```python
from build123d import *

# Parameters (mm, degrees)
F0_W     = 152.4
F0_H     = 152.4
F0_R     = 5.159375
F0_R_2   = 6.35
F0_R_3   = 44.45
F1_DEPTH = 12.7


with BuildPart() as f1:
    # F0 (on Top) → F1 (new body)
    with BuildSketch(Plane.XY):
        Rectangle(F0_W, F0_H)
        with Locations((0, -62.4967)):
            Circle(F0_R, mode=Mode.SUBTRACT)
        with Locations((45.960951, -45.960951)):
            Circle(F0_R_2, mode=Mode.SUBTRACT)
        with Locations((-62.4967, 0)):
            Circle(F0_R, mode=Mode.SUBTRACT)
        with Locations((-45.960951, 45.960951)):
            Circle(F0_R_2, mode=Mode.SUBTRACT)
        Circle(F0_R_3, mode=Mode.SUBTRACT)
        with Locations((62.4967, 0)):
            Circle(F0_R, mode=Mode.SUBTRACT)
        with Locations((0, 62.4967)):
            Circle(F0_R, mode=Mode.SUBTRACT)
    extrude(amount=F1_DEPTH)


solid = f1.part
```
Design review of the part built by this model. Coordinates are the model's own, in mm. Coordinates: 2 decimals unless noted, no trailing zeros. Order: outer loops, then holes, each group sorted by start corner. A loop starts at its lowest first (then second) coordinate and runs counter-clockwise, first axis right, second up. Notation, with made-up numbers: (31, -9) -> (75, -9) arc R24 cw to (75, 19) -> close; hole circle Ø10 at (63, -4). An arc over 180 degrees is marked (long way). One line per item, written item: value. Start each with the question number.
Q1. Take a section at D-D, the plane z = 6.5. State the section outline as (x, y) points, then the cut area to 3 significant figures.
Q2. Mouldability with a two-part tool opening along Y and no side actions: class faces 1 (the cylindrical face through (-0.67, -57.38, 6.26)), 2 (the flat face through (-1, 76.2, 6)), 3 (the cylindrical face through (42.397, 13.352, 6.261)), 4 (the flat face through (-35, 35, 12.7)) as pulls with the +Y half, pulls with the -Y half, needs draft (parallel to the pull), parting line crosses it, or undercut.
Q3. Take a section at A-A, the plane y = 0. State the section outline as (x, z) points.
Q4. Take a section at B-B, the plane x = 23.5. State the section outline as (y, z) points.
Q5. For probe 1 along Y at (x, z) = (0, 9); probe 2 along Y at (x, z) = (3, 10.75); probe 3 along Y at (x, z) = (41, 9.25), list the stretches that pass through material, from the lowest coordinate up.
Values follow:
1. outline: (-76.2, -76.2) -> (76.2, -76.2) -> (76.2, 76.2) -> (-76.2, 76.2) -> close; hole circle Ø10.32 at (-62.5, 0); hole circle Ø12.7 at (-45.96, 45.96); hole circle Ø88.9 at (0, 0); hole circle Ø10.32 at (0, -62.5); hole circle Ø10.32 at (0, 62.5); hole circle Ø12.7 at (45.96, -45.96); hole circle Ø10.32 at (62.5, 0)
1. area: 16,400 mm2
2. face 1: undercut
2. face 2: pulls with the +Y half
2. face 3: undercut
2. face 4: needs draft
3. outline: (-76.2, 0) -> (-67.66, 0) -> (-67.66, 12.7) -> (-76.2, 12.7) -> close; (-57.34, 0) -> (-44.45, 0) -> (-44.45, 12.7) -> (-57.34, 12.7) -> close; (44.45, 0) -> (57.34, 0) -> (57.34, 12.7) -> (44.45, 12.7) -> close; (67.66, 0) -> (76.2, 0) -> (76.2, 12.7) -> (67.66, 12.7) -> close
4. outline: (-76.2, 0) -> (-37.73, 0) -> (-37.73, 12.7) -> (-76.2, 12.7) -> close; (37.73, 0) -> (76.2, 0) -> (76.2, 12.7) -> (37.73, 12.7) -> close
5. probe 1: y = -76.2 to -67.66, -57.34 to -44.45, 44.45 to 57.34, 67.66 to 76.2
5. probe 2: y = -76.2 to -66.69, -58.3 to -44.35, 44.35 to 58.3, 66.69 to 76.2
5. probe 3: y = -76.2 to -49.92, -42 to -17.17, 17.17 to 76.2
